The model under review builds one solid part; all positions refer to its coordinate system, in mm. A direction names the side the tool comes from. Round coordinates to 2 decimals unless told otherwise and drop trailing zeros. Order: outer loops, then holes, each group sorted by start corner. A loop starts at its lowest first (then second) coordinate and runs counter-clockwise, first axis right, second up. Notation, with made-up numbers: M 2,-6 L 60,-6 A8 ccw 60,-1 Z; hole C -10,27 d1. An arc over 180 degrees is marked long. Answer as a JSON object with one key per item and string values. Group by question number.
1) To check wall thickness, follow line 1 (X direction, y = -30, z = 18); line 2 (X direction, y = -18, z = 18); line 3 (Y direction, x = -13, z = 9.5). State the ranges of each line that lie inside material, in increasing order.
2) Consider section B-B, the plane y = -19. Write out the cut boundary in (x, z).
3) Consider section A-A, the plane x = -18.6. Write out the cut boundary in (y, z), then the cut area to 3 significant figures.
4) Consider section D-D, the plane y = 14.5. Write out the cut boundary in (x, z), then the cut area to 3 significant figures.
5) Insertion check: pin 1 Ø9 at (x, y) = (-18.6, 7.5) entering from -Z; pin 2 Ø10 at (y, z) = (-28, 11) entering from +X; pin 3 Ø1.9 at (x, y) = (19.5, -29) entering from +Z. Each pin has a flat end and moves straight along its axis. Give the tip position at first contact, or say it passes through.
6) The part is to be moulded in two halves that separate along Y. For faces 1 (the flat face through (0, -22.9, 26)), 2 (the flat face through (0, 22.9, 14)), 3 (the flat face through (-7, 0, 28.3)), say which applies: +Y half, -Y half, draft (parallel to the pull), parting line (faces both ways), or undercut.
7) Consider section C-C, the plane z = 26. Write out the cut boundary in (x, y).
8) For faces 4 (the cylindrical face through (-11.9, -23.41, 2.78)), 5 (the flat face through (0, 20.5, 12)), 6 (the cylindrical face through (-19.407, 21.717, 9.714)), 7 (the flat face through (-17.75, -27, 14)), list the 3-axis set-ups (+Z, -Z, +X, -X, +Y, -Y) from which the entire face can be reached by the end or side of a thin tool; tool diameter is ignored.
```python
from build123d import *

# Parameters (mm, degrees)
F5_W         = 64
F5_H         = 45.8
F5_W_2       = 59.2
F5_H_2       = 41
F6_DEPTH     = 24.7
F7_W         = 64
F7_H         = 45.8
F7_W_2       = 59.2
F7_H_2       = 41
F8_DEPTH     = 3.6
F9_R         = 5
F10_DEPTH    = 3.1
F11_R        = 14.82
F11_R_2      = 12.42
F12_DEPTH    = 4
F13_DEPTH    = 3.1
F14_R        = 5
F15_DEPTH    = 2.4
F17_R        = 1.75
F18_DEPTH    = 2.4
F20_DEPTH    = 2.4
F22_DEPTH    = 2.4
F23_R        = 1.75
F24_REACH    = 60.9944299909
F25_R        = 0.5
F26_W        = 18
F26_H        = 2.4
F27_DEPTH    = 24.7
F28_R        = 3.75
F29_REACH    = 64.2512842404
F31_DEPTH    = 2.4
F32_T1_DEPTH = 2.4


# Not quite as in the source:
# - a fillet or chamfer that OpenCascade refuses, or shapes differently, is made with other operations: its cross-section is extruded or revolved along the edge and cut away or added
# - a feature names something its author has since deleted; it is built from what else it names


with BuildPart() as f6:
    # F5 (on Top) → F6 (new body)
    with BuildSketch(Plane.XY):
        Rectangle(F5_W, F5_H)
        Rectangle(F5_W_2, F5_H_2, mode=Mode.SUBTRACT)
    extrude(amount=F6_DEPTH)

    # F7 (on face) → F8 (join)
    with BuildSketch(Plane.XY.offset(24.7)):
        Rectangle(F7_W, F7_H)
        Rectangle(F7_W_2, F7_H_2, mode=Mode.SUBTRACT)
        Rectangle(F7_W_2, F7_H_2)
    extrude(amount=F8_DEPTH)

    # F9 (on face) → F10 (cut)
    with BuildSketch(Plane.XY.offset(28.3)):
        with Locations((-18.6, 7.5)):
            Circle(F9_R)
    extrude(amount=-F10_DEPTH, mode=Mode.SUBTRACT)

    # F11 (on face) → F12 (join)
    with BuildSketch(Plane.XY.offset(28.3)):
        with Locations((13.926, 5.264)):
            Circle(F11_R)
        with Locations((13.926, 5.264)):
            Circle(F11_R_2, mode=Mode.SUBTRACT)
    extrude(amount=F12_DEPTH)

    # F13 (cut): a face of the model
    f13_faces = [f6.faces().sort_by_distance(p)[0] for p in [
        (13.926, 5.264, 28.3),
    ]]
    extrude(f13_faces, amount=-F13_DEPTH, mode=Mode.SUBTRACT)

    # F14 (on face) → F15 (cut)
    with BuildSketch(Plane(origin=(0, 22.9, 0), x_dir=(-1, 0, 0), z_dir=(0, 1, 0))):
        with Locations((17.1, 14.15)):
            Circle(F14_R)
    extrude(amount=-F15_DEPTH, mode=Mode.SUBTRACT)

    # F17 (on face) → F18 (join)
    with BuildSketch(Plane(origin=(0, -15.3661306411, -10.759480508), x_dir=(-1, 0, 0), z_dir=(0, 0.8191520443, 0.5735764364))):
        Polygon((0, 24.1349003924), (0, 13.1349003924), (17.75, 13.1349003924), (17.75, 35.1349003924), (0, 35.1349003924), align=None)
        with Locations((13.25, 30.1349003924)):
            Circle(F17_R, mode=Mode.SUBTRACT)
        Polygon((-17.75, 13.1349003924), (0, 13.1349003924), (0, 24.1349003924), (0, 35.1349003924), (-17.75, 35.1349003924), align=None)
        with Locations((-13.25, 30.1349003924)):
            Circle(F17_R, mode=Mode.SUBTRACT)
    extrude(amount=F18_DEPTH)

    # F19 (on face) → F20 (join)
    with BuildSketch(Plane(origin=(-17.75, 0, 0), x_dir=(0, -1, 0), z_dir=(-1, 0, 0))):
        Polygon((22.9, 0), (35.5186815997, 18.0213449744), (33.5527166934, 19.3979284216), (22.9, 19.3979284216), align=None)
    extrude(amount=F20_DEPTH)

    # F21 (on face) → F22 (join)
    with BuildSketch(Plane.YZ.offset(17.75)):
        Polygon((-35.5186815997, 18.0213449744), (-22.9, 0), (-22.9, 19.3979284216), (-33.5527166934, 19.3979284216), align=None)
    extrude(amount=F22_DEPTH)

    f24_end = f6.faces().sort_by_distance((0, 0, 24.7))[0]
    # F23 (on face) → F24 (cut, up to a face of the model that its end follows)
    with BuildSketch(Plane(origin=(0, -15.3661306411, -10.759480508), x_dir=(1, 0, 0), z_dir=(0, -0.8191520443, -0.5735764364))):
        with Locations((-13.25, 30.1349003924)):
            Circle(F23_R)
        with Locations((13.25, 30.1349003924)):
            Circle(F23_R)
    f24_long = extrude(amount=-F24_REACH, mode=Mode.PRIVATE)
    add(split(f24_long, bisect_by=f24_end, keep=Keep.TOP, mode=Mode.PRIVATE), mode=Mode.SUBTRACT)

    # F25
    f25_edges = [f6.edges().sort_by_distance(p)[0] for p in [
        (-32, 0, 28.3),
        (0, -22.9, 28.3),
        (32, 0, 28.3),
        (0, 22.9, 28.3),
        (-23.6, 7.5, 28.3),
        (32, 0, 0),
        (0, 22.9, 0),
        (-32, 22.9, 14.15),
        (-32, 0, 0),
        (-32, -22.9, 14.15),
        (32, -22.9, 14.15),
    ]]
    fillet(f25_edges, radius=F25_R)

    # F26 (on face) → F27 (cut, through all)
    with BuildSketch(Plane(origin=(0, 0, 0), x_dir=(1, 0, 0), z_dir=(0, 0, -1))):
        with Locations((0, 21.7)):
            Rectangle(F26_W, F26_H)
    extrude(amount=-F27_DEPTH, mode=Mode.SUBTRACT)

    f29_end = Plane(origin=(0, -0.3794689119, 24.7), x_dir=(-1, 0, 0), z_dir=(0, 0, -1))
    # F28 (on face) → F29 (cut, up to a plane its end follows)
    with BuildSketch(Plane(origin=(0, -13.4001657348, -9.3828970608), x_dir=(-1, 0, 0), z_dir=(0, 0.8191520443, 0.5735764364))):
        with Locations((13.25, 30.1349003924)):
            Circle(F28_R)
        with Locations((-13.25, 30.1349003924)):
            Circle(F28_R)
    f29_long = extrude(amount=F29_REACH, mode=Mode.PRIVATE)
    add(split(f29_long, bisect_by=f29_end, keep=Keep.TOP, mode=Mode.PRIVATE), mode=Mode.SUBTRACT)

    # F30 (on face) → F31 (cut)
    with BuildSketch(Plane(origin=(0, -15.3661306411, -10.759480508), x_dir=(1, 0, 0), z_dir=(0, -0.8191520443, -0.5735764364))):
        Polygon((-12.5, 27.1349003924), (-12.5, 15.1349003924), (0, 15.1349003924), (12.5, 15.1349003924), (12.5, 27.1349003924), align=None)
    extrude(amount=-F31_DEPTH, mode=Mode.SUBTRACT)

    # F32: fillet of radius 2 on 2 edges, made by hand

    # F32_s2 → F32_t1 (join)
    with BuildSketch(Plane(origin=(0, -15.3661306411, -10.759480508), x_dir=(1, 0, 0), z_dir=(0, 0.8191520443, 0.5735764364))):
        with BuildLine():
            ThreePointArc((-10.5, -15.1349003924), (-11.9142135624, -15.7206868301), (-12.5, -17.1349003924))
            Line((-12.5, -17.1349003924), (-12.5, -15.1349003924))
            Line((-12.5, -15.1349003924), (-10.5, -15.1349003924))
        make_face()
        with BuildLine():
            ThreePointArc((12.5, -17.1349003924), (11.9142135624, -15.7206868301), (10.5, -15.1349003924))
            Line((10.5, -15.1349003924), (12.5, -15.1349003924))
            Line((12.5, -15.1349003924), (12.5, -17.1349003924))
        make_face()
    extrude(amount=F32_T1_DEPTH)


solid = f6.part
```
Results list:
{
 "1": {"line 1": "-20.15 to -17.75, 17.75 to 20.15", "line 2": "-32 to -29.6, 29.6 to 32", "line 3": "-29.55 to -26.62, -22.9 to -20.5, 20.5 to 22.9"},
 "2": {"outline": "M -32,0.5 A0.5 ccw -31.5,0 L -29.6,0 L -29.6,24.7 L 29.6,24.7 L 29.6,0 L 31.5,0 A0.5 ccw 32,0.5 L 32,27.8 A0.5 ccw 31.5,28.3 L -31.5,28.3 A0.5 ccw -32,27.8 Z"},
 "3": {"outline": "M -35.52,18.02 L -22.9,0 L -20.5,0 L -20.5,24.7 L 20.5,24.7 L 20.5,18.92 L 22.9,18.92 L 22.9,27.8 A0.5 ccw 22.4,28.3 L 13,28.3 A0.5 ccw 12.5,27.8 L 12.5,25.2 L 2.5,25.2 L 2.5,27.8 A0.5 ccw 2,28.3 L -22.4,28.3 A0.5 ccw -22.9,27.8 L -22.9,19.4 L -33.55,19.4 Z; M 20.5,0 L 22.4,0 A0.5 ccw 22.9,0.5 L 22.9,9.38 L 20.5,9.38 Z", "area": "359 mm^2"},
 "4": {"outline": "M -32,0.5 A0.5 ccw -31.5,0 L -29.6,0 L -29.6,24.7 L 29.6,24.7 L 29.6,0 L 31.5,0 A0.5 ccw 32,0.5 L 32,27.8 A0.5 ccw 31.5,28.3 L 25.52,28.3 L 25.52,32.3 L 22.23,32.3 L 22.23,25.2 L 5.62,25.2 L 5.62,32.3 L 2.34,32.3 L 2.34,28.3 L -31.5,28.3 A0.5 ccw -32,27.8 Z", "area": "324 mm^2"},
 "5": {"pin 1": "z = 24.7", "pin 2": "x = 20.15", "pin 3": "z = 19.4"},
 "6": {"face 1": "undercut", "face 2": "+Y half", "face 3": "draft"},
 "7": {"outline": "M -32,-22.4 A0.5 ccw -31.5,-22.9 L 31.5,-22.9 A0.5 ccw 32,-22.4 L 32,22.9 L -31.5,22.9 A0.5 ccw -32,22.4 Z; hole C -18.6,7.5 d10; hole C 13.93,5.26 d24.84"},
 "8": {"face 4": "-Y", "face 5": "-Z", "face 6": "+Y", "face 7": "+Z"}
}
